```python
from build123d import *

# Parameters (mm, degrees)
SKETCH_W        = 155
SKETCH_H        = 40
PAD_DEPTH       = 3
SKETCH001_W     = 20
SKETCH001_H     = 3
SKETCH001_W_2   = 29
POCKET_DEPTH    = 3.001
SKETCH002_W     = 3
SKETCH002_H     = 10
POCKET001_DEPTH = 323.213429


with BuildPart() as part:
    # Sketch → Pad (new body)
    with BuildSketch(Plane.XZ):
        Rectangle(SKETCH_W, SKETCH_H)
    extrude(amount=PAD_DEPTH)

    # Sketch001 (on Face6 of Pad) → Pocket (cut, through all)
    with BuildSketch(Plane.XZ.offset(3)):
        with Locations((64.5, -13.5)):
            Rectangle(SKETCH001_W, SKETCH001_H)
        with Locations((24.5, -13.5)):
            Rectangle(SKETCH001_W, SKETCH001_H)
        with Locations((-15.5, -13.5)):
            Rectangle(SKETCH001_W, SKETCH001_H)
        with Locations((-60, -13.5)):
            Rectangle(SKETCH001_W_2, SKETCH001_H)
    extrude(amount=-POCKET_DEPTH, mode=Mode.SUBTRACT)

    # Sketch002 (on Face5 of Pocket) → Pocket001 (cut, through all)
    with BuildSketch(Plane.XZ.offset(3)):
        with Locations((-76, 15)):
            Rectangle(SKETCH002_W, SKETCH002_H)
        with Locations((-76, -5)):
            Rectangle(SKETCH002_W, SKETCH002_H)
    pocket001 = extrude(amount=-POCKET001_DEPTH, mode=Mode.SUBTRACT)

    # Mirrored: Pocket001 across Sketch002 V_Axis
    add(pocket001.mirror(Plane(origin=(0, -3, 0), x_dir=(0, -1, 0), z_dir=(1, 0, 0))), mode=Mode.SUBTRACT)


solid = part.part
```
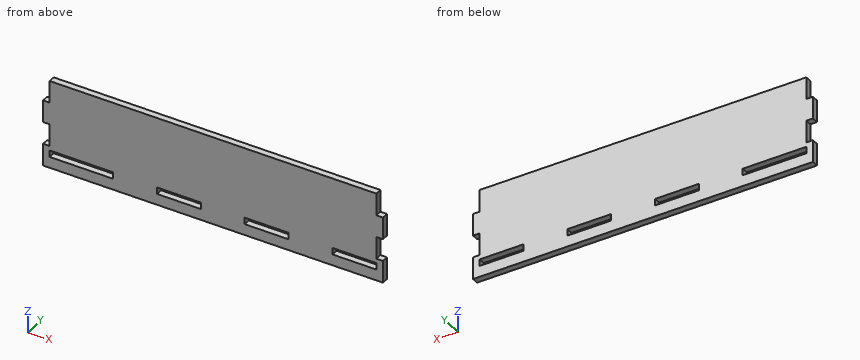
Model file for the job. Use its own axes, mm. Give positions to 0.01 mm unless a question says otherwise; leave off trailing zeros. Loops run counter-clockwise (first coordinate to the right, second up) from the corner with the lowest first, then second, coordinate; pieces in that order, holes last. Notation, with made-up numbers: (19.25, -25.75) -> (71.25, -25.75) arc R12 cw to (71.25, -6.75) -> close; hole circle Ø11 at (44.25, 53). An arc over 180 degrees is marked (long way). Use CSV: the item, a comma, the result in double quotes. Start each with the question number.
1) Slice it at B-B on y = -1.65. Give the number of separate pieces and of enclosed holes in the cut face, plus the area to 3 significant figures.
2) Flat gauge pins, fed straight in: pin 1 Ø0.9 at (x, y) = (-75.5, -1.5) entering from +Z; pin 2 Ø0.9 at (y, z) = (-1.5, -3) entering from +X; pin 3 Ø0.9 at (y, z) = (-1.5, 15.5) entering from -X. Where does each tip first touch, or does it go through?
3) Slice it at A-A on x = 64. Give the cut face in (y, z), plus the area to 3 significant figures.
4) Slice it at C-C on z = 16. Give the cut face in (x, y).
5) Wall check: line 1 (Z direction, x = -70.5, y = -1.2); line 2 (X direction, y = -0.6, z = -14); line 3 (X direction, y = -2.8, z = -2). Give the ranges that are in metal, low to high.
Computed values:
1,separate pieces,"1"
1,enclosed holes,"4"
1,area,"5,810 mm^2"
2,pin 1,"stops at z = 10"
2,pin 2,"stops at x = 74.5"
2,pin 3,"stops at x = -74.5"
3,outline,"(-3, -20) -> (0, -20) -> (0, -15) -> (-3, -15) -> close; (-3, -12) -> (0, -12) -> (0, 20) -> (-3, 20) -> close"
3,area,"111 mm^2"
4,outline,"(-74.5, -3) -> (74.5, -3) -> (74.5, 0) -> (-74.5, 0) -> close"
5,line 1,"z = -20 to -15, -12 to 20"
5,line 2,"x = -77.5 to -74.5, -45.5 to -25.5, -5.5 to 14.5, 34.5 to 54.5, 74.5 to 77.5"
5,line 3,"x = -74.5 to 74.5"
